Work out the finished part from the listing and answer in its coordinate system (mm). Give positions to 0.01 mm unless a question says otherwise; leave off trailing zeros. Order: outer loops, then holes, each group sorted by start corner. A loop starts at its lowest first (then second) coordinate and runs counter-clockwise, first axis right, second up. Notation, with made-up numbers: (36.25, -31) - (86.25, -31) arc R18 ccw to (86.25, 1) - close; hole circle Ø2 at (75, 9). An arc over 180 degrees is marked (long way). Return JSON: item names as keys, results as strings. Group by question number.
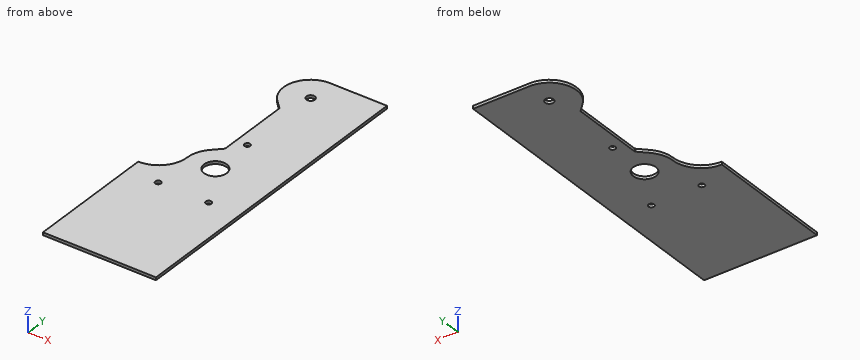
from build123d import *

# Parameters (mm, degrees)
F0_W     = 127
F0_H     = 252.73
F1_DEPTH = 3.175
F2_R     = 12.7
F2_R_2   = 3.175
F2_R_3   = 4.7625
F3_DEPTH = 3.176
F4_W     = 127
F4_H     = 3.175
F5_DEPTH = 101.6


with BuildPart() as f1:
    # F0 (on Top) → F1 (new body)
    with BuildSketch(Plane.XY):
        Rectangle(F0_W, F0_H)
    extrude(amount=F1_DEPTH)

    # F2 (on face) → F3 (cut, through all)
    with BuildSketch(Plane.XY.offset(3.175)):
        with BuildLine():
            Line((-12.7, 65.405), (-21.59, 74.295))
            ThreePointArc((-21.59, 74.295), (-28.540289, 106.734338), (-1.796051, 126.365))
            Line((-1.796051, 126.365), (-63.5, 126.365))
            Line((-63.5, 126.365), (-63.5, 116.205))
            Line((-63.5, 116.205), (-63.5, -69.215))
            Line((-63.5, -69.215), (-63.5, -81.915))
            ThreePointArc((-63.5, -81.915), (-41.04936, -72.61564), (-31.75, -50.165))
            ThreePointArc((-31.75, -50.165), (-29.333175, -38.014801), (-22.45064, -27.71436))
            Line((-22.45064, -27.71436), (-12.7, -17.963719))
            Line((-12.7, -17.963719), (-12.7, 65.405))
        make_face()
        with Locations((0, -50.165)):
            Circle(F2_R)
        with Locations((28.3845, -99.219948)):
            Circle(F2_R_2)
        with Locations((-28.3845, -99.219948)):
            Circle(F2_R_2)
        with Locations((0, -1.110052)):
            Circle(F2_R_2)
        with Locations((0, 95.885)):
            Circle(F2_R_3)
    extrude(amount=-F3_DEPTH, mode=Mode.SUBTRACT)

    # F4 (on face) → F5 (join)
    with BuildSketch(Plane.XZ.offset(126.365)):
        with Locations((0, 1.5875)):
            Rectangle(F4_W, F4_H)
    extrude(amount=F5_DEPTH)


solid = f1.part
1. The part is cut by section A-A (z = 2.3). State how many separate pieces and enclosed holes the cut face has, and give its area (3 significant figures).
2. Each of these flat-tipped pins is pushed along its axis until it touches: pin 1 (1 mm diameter, centred on y = 7.5, z = 2, fed in from -X); pin 2 (1.5 mm diameter, centred on x = -36.5, z = 2.5, fed in from +Y); pin 3 (20.5 mm diameter, centred on x = 0, y = -50.165, fed in from -Z); pin 4 (1.5 mm diameter, centred on y = -66, z = 0.5, fed in from -X). Where does it stop, or does it pass through?
3. Consider probe 1 along Y at (x, z) = (0, 2.35) (1 decimal); probe 2 along Y at (x, z) = (1, 2.85) (3 decimals); probe 3 along Y at (x, z) = (-4, 1.9) (3 decimals). Determine where each line is inside the solid, lowest interval first. Write a range as from..to.
4. The part is cut by section B-B (x = -37.5). Give the vertices of the cut face in (y, z) (3 decimals).
Answers:
{
 "1": {"separate pieces": "1", "enclosed holes": "5", "area": "35,700 mm^2"},
 "2": {"pin 1": "stops at x = -12.7", "pin 2": "stops at y = -65.59", "pin 3": "passes through", "pin 4": "stops at x = -36.43"},
 "3": {"probe 1": "y = -228..-62.9, -37.5..-4.3, 2.1..91.1, 100.6..126.4", "probe 2": "y = -227.965..-62.826, -37.504..-4.123, 1.903..91.229, 100.541..126.365", "probe 3": "y = -227.965..-62.219, -38.111..93.3, 98.47..126.155"},
 "4": {"outline": "(-227.965, 0) - (-68.388, 0) - (-68.388, 3.175) - (-227.965, 3.175) - close"}
}
